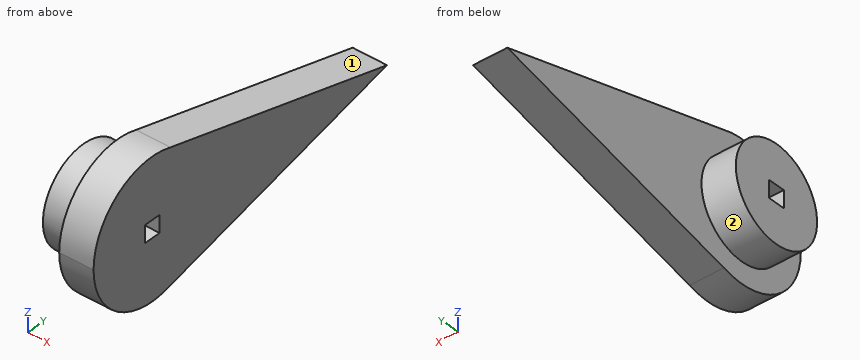
```python
from build123d import *

# Parameters (mm, degrees)
F1_DEPTH = 6.35
F2_W     = 3.175
F2_H     = 3.175
F3_DEPTH = 25.4
F4_R     = 8.794705
F4_W     = 3.175
F4_H     = 3.175
F5_DEPTH = 6.35


with BuildPart() as f1:
    # F0 (on Right) → F1 (new body)
    with BuildSketch(Plane.YZ):
        with BuildLine():
            Line((50.8, 0), (3.935791, 12.074749))
            ThreePointArc((3.935791, 12.074749), (-7.460076, 10.277999), (-12.7, 0))
            ThreePointArc((-12.7, 0), (-7.460076, -10.277999), (3.935791, -12.074749))
            Line((3.935791, -12.074749), (50.8, 0))
        make_face()
    extrude(amount=F1_DEPTH)

    # F2 (on face) → F3 (cut)
    with BuildSketch(Plane.YZ.offset(6.35)):
        Rectangle(F2_W, F2_H)
    extrude(amount=-F3_DEPTH, mode=Mode.SUBTRACT)

    # F4 (on Right) → F5 (join)
    with BuildSketch(Plane.YZ):
        Circle(F4_R)
        Rectangle(F4_W, F4_H, mode=Mode.SUBTRACT)
    extrude(amount=-F5_DEPTH)


solid = f1.part
```
Build history of the part. All positions in model axes, mm. Face numbers are marked on the shaded views. A direction names the side the tool comes from. Coordinates: 2 decimals unless noted, no trailing zeros. Order: outer loops, then holes, each group sorted by start corner. A loop starts at its lowest first (then second) coordinate and runs counter-clockwise, first axis right, second up. Notation, with made-up numbers: (49.5, 84.5) -> (62.5, 84.5) arc R17 ccw to (62.5, 115.5) -> close; hole circle Ø9 at (-10, 11.5). An arc over 180 degrees is marked (long way). Answer in a Markdown table with one row per item. Add a question column.
Q1. Band-saw the part on D-D, the plane x = -3.5. List the corners of the cut face in (y, z), then the cut area to 3 significant figures.
Q2. Drop flat-ended pins along their axis: pin 1 (12 mm diameter, centred on y = 17, z = -6, fed in from -X); pin 2 (1 mm diameter, centred on x = 2, z = -0.5, fed in from -Y); pin 3 (6 mm diameter, centred on x = 1, z = -6.5, fed in from -Y); pin 4 (6 mm diameter, centred on x = -1, z = -4, fed in from -Y). Give the stop position or say it passes through.
Q3. Band-saw the part on C-C, the plane z = 3.75. List the corners of the cut face in (x, y).
Q4. Band-saw the part on B-B, the plane x = 5.25. List the corners of the cut face in (y, z), then the cut area to 3 significant figures.
Q5. Band-saw the part on A-A, the plane y = 0. List the corners of the cut face in (x, z).
Q6. Wall check: line 1 along Y through (x, z) = (-4.75, -0.5); line 2 along Z through (x, y) = (3, 41) (3 decimals); line 3 along Z through (x, y) = (0.25, 35.5). Give the ranges that are in metal, low to high. Write a range as [from, to].
Q7. Which spindle directions (+Z, -Z, +X, -X, +Y, -Y) get a long thin tool onto all of the face, cutting with end or side? Do the marked faces 1 and 2. Say none if no direction does.
Answers follow:
| question | item | result |
|---|---|---|
| 1 | outline | circle Ø17.59 at (0, 0); hole (-1.59, -1.59) -> (1.59, -1.59) -> (1.59, 1.59) -> (-1.59, 1.59) -> close |
| 1 | area | 233 mm^2 |
| 2 | pin 1 | x = 0 |
| 2 | pin 2 | y = -12.7 |
| 2 | pin 3 | y = -12.21 |
| 2 | pin 4 | y = -12.65 |
| 3 | outline | (-6.35, -7.96) -> (0, -7.96) -> (0, -12.13) -> (6.35, -12.13) -> (6.35, 36.25) -> (0, 36.25) -> (0, 7.96) -> (-6.35, 7.96) -> close |
| 4 | outline | (-12.7, 0) arc R12.7 ccw to (3.94, -12.07) -> (50.8, 0) -> (3.94, 12.07) arc R12.7 ccw to start; hole (-1.59, -1.59) -> (1.59, -1.59) -> (1.59, 1.59) -> (-1.59, 1.59) -> close |
| 4 | area | 907 mm^2 |
| 5 | outline | (-6.35, -8.79) -> (0, -8.79) -> (0, -12.7) -> (6.35, -12.7) -> (6.35, -1.59) -> (-6.35, -1.59) -> close; (-6.35, 1.59) -> (6.35, 1.59) -> (6.35, 12.7) -> (0, 12.7) -> (0, 8.79) -> (-6.35, 8.79) -> close |
| 6 | line 1 | [-8.78, -1.59], [1.59, 8.78] |
| 6 | line 2 | [-2.525, 2.525] |
| 6 | line 3 | [-3.94, 3.94] |
| 7 | face 1 | +Z, +X, -X, +Y |
| 7 | face 2 | -X |
